Build history of the part. All positions in model axes, mm. Face numbers are marked on the shaded views. A direction names the side the tool comes from. Give positions to 0.01 mm unless a question says otherwise; leave off trailing zeros. Order: outer loops, then holes, each group sorted by start corner. A loop starts at its lowest first (then second) coordinate and runs counter-clockwise, first axis right, second up. Notation, with made-up numbers: (61, -18) - (116, -18) arc R8 ccw to (116, -14) - close; hole circle Ø4 at (73, -26). An arc over 180 degrees is marked (long way). Use a Markdown table: item, result.
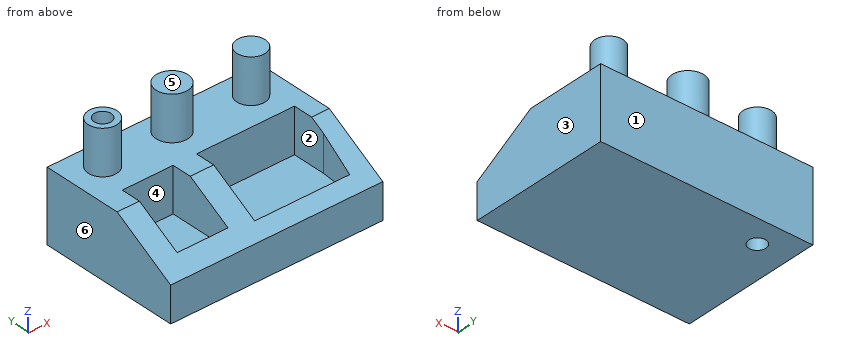
from build123d import *

# Parameters (mm, degrees)
F0_W     = 120
F0_H     = 80
F1_DEPTH = 40
F2_W     = 28.798189
F2_H     = 35.557579
F3_DEPTH = 25
F5_DEPTH = 120.001
F6_R     = 8.123016
F6_R_2   = 9.029606
F6_R_3   = 7.997109
F7_DEPTH = 25
F8_R     = 4.835396
F9_DEPTH = 65.001


with BuildPart() as f1:
    # F0 (on Top) → F1 (new body)
    with BuildSketch(Plane.XY):
        with Locations((-4.226902, -5.768067)):
            Rectangle(F0_W, F0_H)
    extrude(amount=F1_DEPTH)

    # F2 (on face) → F3 (cut)
    with BuildSketch(Plane.XY.offset(40)):
        with Locations((-37.26047, -17.778789)):
            Rectangle(F2_W, F2_H)
        Polygon((45.773098, 0), (-9.63674, 0), (-9.63674, -37.675409), (44.113688, -37.675409), (45.773098, -18.742215), align=None)
    extrude(amount=-F3_DEPTH, mode=Mode.SUBTRACT)

    # F4 (on face) → F5 (cut, through all)
    with BuildSketch(Plane.YZ.offset(55.773098)):
        Polygon((-45.768067, 40), (-45.768067, 20), (-11.09978, 40), align=None)
    extrude(amount=-F5_DEPTH, mode=Mode.SUBTRACT)

    # F6 (on face) → F7 (join)
    with BuildSketch(Plane.XY.offset(40)):
        with Locations((-46.003349, 19.200161)):
            Circle(F6_R)
        with Locations((-6.039798, 20.013448)):
            Circle(F6_R_2)
        with Locations((37.330549, 18.490579)):
            Circle(F6_R_3)
    extrude(amount=F7_DEPTH)

    # F8 (on face) → F9 (cut, through all)
    with BuildSketch(Plane.XY.offset(65)):
        with Locations((-46.003349, 19.200161)):
            Circle(F8_R)
    extrude(amount=-F9_DEPTH, mode=Mode.SUBTRACT)


solid = f1.part
1) Two-plate mould, pull along X, no slides. Class the marked faces 3, 4, 5 and 6: +X half, -X half, draft (parallel to the pull), parting line (faces both ways), or undercut.
Computed:
| item | result |
|---|---|
| face 3 | +X half |
| face 4 | undercut |
| face 5 | draft |
| face 6 | -X half |
2) Pin check, flat tips, straight feed: P1, Ø20, axis at x = 17, z = 31, coming from the -Y side; P2, Ø1.5, axis at x = 32, z = 42, coming from the -Y side; P3, Ø4, axis at x = -45.5, z = 45.5, coming from the -Y side. Stop position of each tip, or through.
Computed:
| item | result |
|---|---|
| P1 | stops at y = -44.03 |
| P2 | stops at y = 11.94 |
| P3 | stops at y = 11.08 |
3) Slice it at B-B (z = 28). Write the cut outline in (x, y).
Computed:
| item | result |
|---|---|
| outline | (-64.23, -31.9) - (-51.66, -31.9) - (-51.66, 0) - (-22.86, 0) - (-22.86, -31.9) - (-9.64, -31.9) - (-9.64, 0) - (45.77, 0) - (45.77, -18.74) - (44.62, -31.9) - (55.77, -31.9) - (55.77, 34.23) - (-64.23, 34.23) - close; hole circle Ø9.67 at (-46, 19.2) |
4) Slice it at C-C (y = -5.5). Write the cut outline in (x, z), and give its area (3 significant figures).
Computed:
| item | result |
|---|---|
| outline | (-64.23, 0) - (55.77, 0) - (55.77, 40) - (45.77, 40) - (45.77, 15) - (-9.64, 15) - (-9.64, 40) - (-22.86, 40) - (-22.86, 15) - (-51.66, 15) - (-51.66, 40) - (-64.23, 40) - close |
| area | 2,690 mm² |
5) Slice it at A-A (x = -24.5). Write the cut outline in (y, z), and give its area (3 significant figures).
Computed:
| item | result |
|---|---|
| outline | (-45.77, 0) - (34.23, 0) - (34.23, 40) - (0, 40) - (0, 15) - (-35.56, 15) - (-35.56, 25.89) - (-45.77, 20) - close |
| area | 2,140 mm² |
6) Wall check: line 1 (X direction, y = -1, z = 26.5); line 2 (Z direction, x = -51.5, y = -18.5); line 3 (Z direction, x = 6, y = 14.5). Give the ranges that are in metal, low to high. Write a range as from..to.
Computed:
| item | result |
|---|---|
| line 1 | x = -64.23..-51.66, -22.86..-9.64, 45.77..55.77 |
| line 2 | z = 0..15 |
| line 3 | z = 0..40 |
7) Slice it at D-D (x = 16). Write the cut outline in (y, z), and give its area (3 significant figures).
Computed:
| item | result |
|---|---|
| outline | (-45.77, 0) - (34.23, 0) - (34.23, 40) - (0, 40) - (0, 15) - (-37.68, 15) - (-37.68, 24.67) - (-45.77, 20) - close |
| area | 2,120 mm² |
8) Tool access for the marked faces 1 and 2: list every direction of +Z, -Z, +X, -X, +Y, -Y with a clear straight run to the whole face (end or side of a thin tool).
Computed:
| item | result |
|---|---|
| face 1 | +Z, -Z, +X, -X, +Y |
| face 2 | +Z |
